from build123d import *


# Not quite as in the source:
# - ends of sketch curves that miss each other by under 0.0002 mm in the source are joined


with BuildPart() as f2:
    # F1 (on Top) → F2 (revolve)
    with BuildSketch(Plane.XY):
        with BuildLine():
            ThreePointArc((-1.5543495265, -30.6423329465), (-1.4953949864, -31.3914475732), (-0.835025, -31.75))
            Line((-0.835025, -31.75), (1.984375, -31.75))
            Line((1.984375, -31.75), (1.984375, 31.75))
            Line((1.984375, 31.75), (-1.984375, 31.75))
            Line((-1.984375, 31.75), (-1.984375, -26.7380212))
            Line((-1.984375, -26.7380212), (-0.5228082, -27.3887438))
            ThreePointArc((-0.5228082, -27.3887438), (-0.322079197, -27.6002624898), (-0.3297130763, -27.8917673251))
            Line((-0.3297130763, -27.8917673251), (-1.5543495265, -30.6423329465))
        make_face()
    revolve(axis=Axis((1.984375, 0, 0), (0, -1, 0)))


solid = f2.part
For this review, take the finished solid that the model builds, in its own axes (mm). Round coordinates to 2 decimals unless told otherwise and drop trailing zeros. Loops run counter-clockwise (first coordinate to the right, second up) from the corner with the lowest first, then second, coordinate; pieces in that order, holes last. Notation, with made-up numbers: (-8.75, 12) - (1.25, 12) arc R4 cw to (1.25, 17) - close; hole circle Ø8 at (88.25, 23). An arc over 180 degrees is marked (long way). One line per item, written item: value. Start each with the question number.
Item 1: For L1, parallel to Y at x = 0.25, z = -2.75; L2, parallel to Y at x = 4.75, z = -1.75; L3, parallel to X at y = 1, z = -0.25, list the stretches that pass through material, from the lowest coordinate up.
Item 2: Clearance check with a flat-ended pin moving along its axis: pin 1 Ø1 at (x, y) = (0.5, 12) entering from +Z. State where the tip first meets the part, or that it passes through.
Item 3: The part is to be moulded in two halves that separate along Y. For faces 1 (the flat face through (2, -31.75, 0)), 2 (the conical face through (-0.296, -28.064, -0.718)), 3 (the cylindrical face through (-1.68, 2.1, 1.52)), 4 (the flat face through (2, 31.75, 0)), say which applies: +Y half, -Y half, draft (parallel to the pull), parting line (faces both ways), or undercut.
Item 4: Take a section at A-A (z = 0). Give the boundary of the cut face in (x, y), plus the area to 3 significant figures.
Item 5: Take a section at B-B (y = 18). Give the boundary of the cut face in (x, z), plus the area to 3 significant figures.
Answer below:
1. L1: y = -31.62 to -30, -27.06 to 31.75
1. L2: y = -31.61 to -30.05, -27.05 to 31.75
1. L3: x = -1.98 to 5.95
2. pin 1: stops at z = 3.84
3. face 1: -Y half
3. face 2: undercut
3. face 3: draft
3. face 4: +Y half
4. outline: (-1.98, -26.74) - (-0.52, -27.39) arc R0.38 cw to (-0.33, -27.89) - (-1.55, -30.64) arc R0.79 ccw to (-0.84, -31.75) - (4.8, -31.75) arc R0.79 ccw to (5.52, -30.64) - (4.3, -27.89) arc R0.38 cw to (4.49, -27.39) - (5.95, -26.74) - (5.95, 31.75) - (-1.98, 31.75) - close
4. area: 495 mm2
5. outline: circle Ø7.94 at (1.98, 0)
5. area: 49.5 mm2
